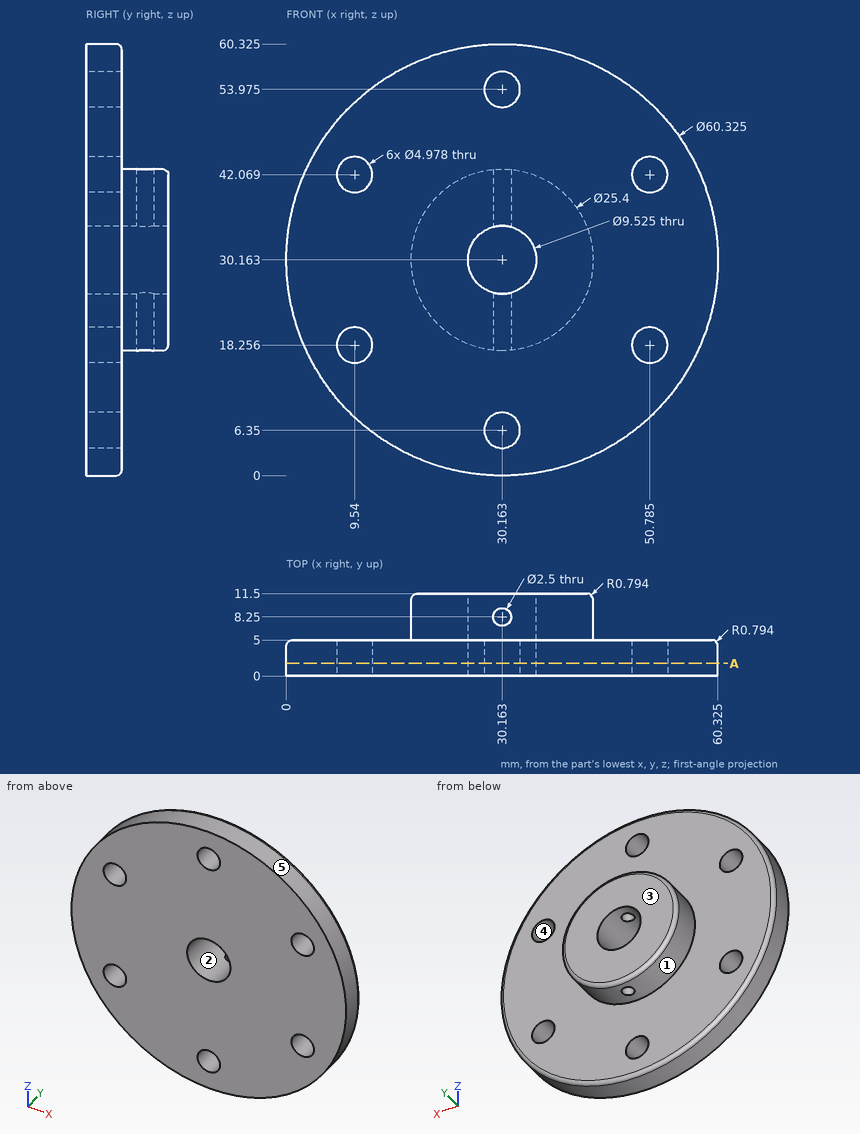
Check sheet for the drawn part. Datum: minimum x, y, z corner. Units: mm. A direction names the side the tool comes from. Give positions to 0.01 mm unless a question says otherwise; leave off trailing zeros. Put each result on its own line as item: value.
1. Set-up check for the marked faces 1 and 2: record each of +Z, -Z, +X, -X, +Y, -Y from which the full face is reachable in a straight line by a thin tool's end or side.
Ans:
face 1: +Y
face 2: +Y, -Y
2. Sectioned sample at A-A, the plane y = 1.75. Give the number of separate pieces and of enclosed holes in the cut face, plus the area to 3 significant figures.
Ans:
separate pieces: 1
enclosed holes: 7
area: 2,670 mm²
3. Draft check along Z on the marked faces 3, 4 and 5. Enter one of: +Z half, -Z half, draft (parallel to the pull), parting line (faces both ways), or undercut.
Ans:
face 3: draft
face 4: undercut
face 5: parting line
4. Thickness scan on line 1 (Y direction, x = 18, z = 42.5); line 2 (Y direction, x = 22.5, z = 21); line 3 (X direction, y = 2.5, z = 28) (1 decimal). Record the ranges inside material, lowest first.
Ans:
line 1: y = 0 to 5
line 2: y = 0 to 11.5
line 3: x = 0.1 to 25.9, 34.4 to 60.2
5. Go/stop test with flat-tipped pins: pin 1 (1.5 mm diameter, centred on y = 4, z = 21, fed in from +X); pin 2 (1.5 mm diameter, centred on y = 7.5, z = 47, fed in from -X); pin 3 (3 mm diameter, centred on x = 30.16, y = 8.25, fed in from -Z); pin 4 (1.5 mm diameter, centred on x = 29, y = 1.5, fed in from +Z). Record where each tip stops, or that it passes through.
Ans:
pin 1: stops at x = 59.13
pin 2: passes through
pin 3: stops at z = 17.46
pin 4: stops at z = 60.32
